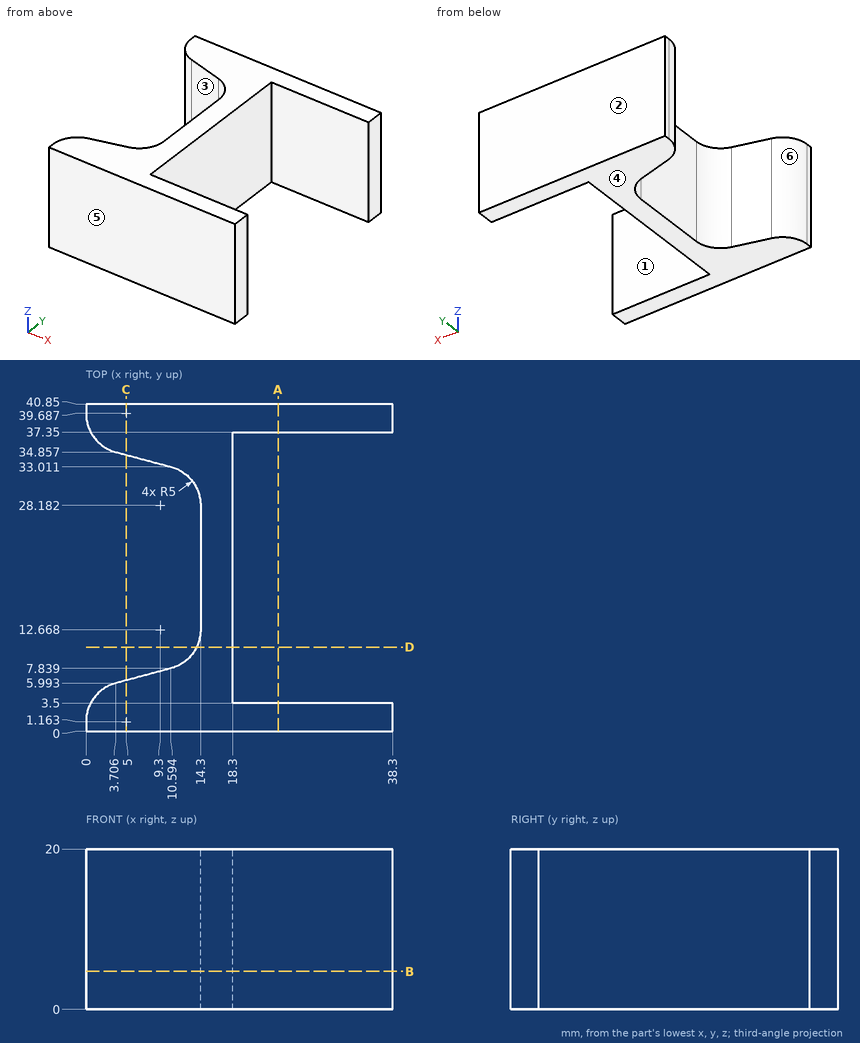
Geometry check sheet. Reference: drawing and pictorial views, mm from the part's lowest x, y, z. A direction names the side the tool comes from. Give positions to 0.01 mm unless a question says otherwise; leave off trailing zeros. Loops run counter-clockwise (first coordinate to the right, second up) from the corner with the lowest first, then second, coordinate; pieces in that order, holes last. Notation, with made-up numbers: (39.5, 7) - (62.5, 7) arc R21 ccw to (62.5, 31) - close; hole circle Ø2 at (65, 42.25). An arc over 180 degrees is marked (long way). One line per question, with ' | ' between items. Start each with the question number.
1. Cross-section at A-A, the plane x = 24. Enter the section's corners in (y, z).
2. Draft check along Y on the marked faces 4, 5 and 6. Enter one of: released by +Y, released by -Y, zero draft, split by the parting line, or undercut.
3. Cross-section at D-D, the plane y = 10.5. Enter the section's corners in (x, z) (1 decimal), plus the area to 3 significant figures.
4. Gauge pin test, flat end, axial feed: pin 1 Ø5 at (y, z) = (16, 15) entering from +X. Record the tip position at first contact, or that the pin passes through.
5. Cross-section at B-B, the plane z = 4.75. Enter the section's corners in (x, y), plus the area to 3 significant figures.
6. Material ranges on line 1 along Y through (x, z) = (33, 3.5); line 2 along Y through (x, z) = (9, 13); line 3 along X through (y, z) = (13.5, 7), recorded low to high. Write a range as [from, to].
7. Cross-section at C-C, the plane x = 5. Enter the section's corners in (y, z), plus the area to 3 significant figures.
8. Set-up check for the marked faces 1, 2 and 3: record each of +Z, -Z, +X, -X, +Y, -Y from which the full face is reachable in a straight line by a thin tool's end or side.
Check result:
1) outline: (0, 0) - (3.5, 0) - (3.5, 20) - (0, 20) - close; (37.35, 0) - (40.85, 0) - (40.85, 20) - (37.35, 20) - close
2) face 4: zero draft | face 5: released by -Y | face 6: undercut
3) outline: (13.8, 0) - (18.3, 0) - (18.3, 20) - (13.8, 20) - close | area: 89.9 mm2
4) pin 1: stops at x = 18.3
5) outline: (0, 0) - (38.3, 0) - (38.3, 3.5) - (18.3, 3.5) - (18.3, 37.35) - (38.3, 37.35) - (38.3, 40.85) - (0, 40.85) - (0, 39.69) arc R5 ccw to (3.71, 34.86) - (10.59, 33.01) arc R5 cw to (14.3, 28.18) - (14.3, 12.67) arc R5 cw to (10.59, 7.84) - (3.71, 5.99) arc R5 ccw to (0, 1.16) - close | area: 501 mm2
6) line 1: y = [0, 3.5], [37.35, 40.85] | line 2: y = [0, 7.41], [33.44, 40.85] | line 3: x = [14.3, 18.3]
7) outline: (0, 0) - (6.34, 0) - (6.34, 20) - (0, 20) - close; (34.51, 0) - (40.85, 0) - (40.85, 20) - (34.51, 20) - close | area: 254 mm2
8) face 1: +Z, -Z, +X | face 2: +Z, -Z, +X, -X, +Y | face 3: +Z, -Z, -X
